Build history of the part. All positions in model axes, mm. A direction names the side the tool comes from. Coordinates: 2 decimals unless noted, no trailing zeros. Order: outer loops, then holes, each group sorted by start corner. A loop starts at its lowest first (then second) coordinate and runs counter-clockwise, first axis right, second up. Notation, with made-up numbers: (42.5, 69.25) - (76.5, 69.25) arc R28 ccw to (76.5, 106.25) - close; hole circle Ø2 at (2, -30.75). An arc over 180 degrees is marked (long way). Write each question's results on one line, items separated by ' | '.
Autodesk Inventor part; units mm, degrees
ref_plane "YZ Plane" through (0, 0, 0) normal (1, 0, 0) x (0, 1, 0)
ref_plane "XZ Plane" through (0, 0, 0) normal (0, 1, 0) x (-1, 0, 0)
ref_plane "XY Plane" through (0, 0, 0) normal (0, 0, 1) x (1, 0, 0)
sketch "Sketch1" plane through (0, 0, 0) normal (0, 1, 0) x (-1, 0, 0)
  circle A0 centre (0, 0) radius 2
  dimension "d0" = 4
extrude "Extrusion1" add sketch "Sketch1" along normal blind 35
sketch "Sketch2" plane through (0, 35, 0) normal (0, 1, 0) x (1, 0, 0)
  circle A0 centre (0, 0) radius 2
  circle A1 centre (0, 0) radius 3.5
  dimension "d3" = 7
extrude "Extrusion2" add sketch "Sketch2" along normal blind 4 contours A0 | A1
sketch "Sketch3" plane through (0, 39, 0) normal (0, 1, 0) x (1, 0, 0)
  circle A0 centre (0, 0) radius 3.5
  line L0 (0, 1.8475) -> (1.6, 0.9238)
  line L1 (1.6, 0.9238) -> (1.6, -0.9238)
  line L2 (1.6, -0.9238) -> (0, -1.8475)
  line L3 (0, -1.8475) -> (-1.6, -0.9238)
  line L4 (-1.6, -0.9238) -> (-1.6, 0.9238)
  line L5 (-1.6, 0.9238) -> (0, 1.8475)
  dimension "d6" = 1.6
extrude "Extrusion3" cut sketch "Sketch3" against normal blind 3 contours L0 L1 L2 L3 L4 L5
thread "Thread1"
chamfer "Chamfer1" distance 0.25 angle 45 1 edges at (2, 0, 0)
properties part number "SHCS4x35"
1. Tool access for faces 1 (the face through (2, 35, 2)), 2 (the face through (3.233, 36.972, -1.341)), 3 (the face through (0.81, 37.52, 1.38)): list every direction of +Z, -Z, +X, -X, +Y, -Y with a clear straight run to the whole face (end or side of a thin tool).
Solved:
face 1: -Y | face 2: +Y, -Y | face 3: +Y
2. Band-saw the part on C-C on x = -3. Give the cut face in (y, z).
Solved:
outline: (35, -1.8) - (39, -1.8) - (39, 1.8) - (35, 1.8) - close
3. Band-saw the part on B-B on y = 9. Give the cut face in (x, z).
Solved:
outline: circle Ø4 at (0, 0)
4. Probe line 1 (Y direction, x = -2.25, z = 1.5); line 2 (Z direction, x = -0.75, y = 11.5); line 3 (Y direction, x = -0.75, z = 1.25). List the from-to ranges inside material, lowest first.
Solved:
line 1: y = 35 to 39 | line 2: z = -1.85 to 1.85 | line 3: y = 0 to 36
5. Band-saw the part on D-D on x = 2.5. Give the cut face in (y, z).
Solved:
outline: (35, -2.45) - (39, -2.45) - (39, 2.45) - (35, 2.45) - close
6. Band-saw the part on A-A on z = 0. Give the cut face in (x, y).
Solved:
outline: (-3.5, 35) - (-2, 35) - (-2, 0.25) - (-1.75, 0) - (1.75, 0) - (2, 0.25) - (2, 35) - (3.5, 35) - (3.5, 39) - (1.6, 39) - (1.6, 36) - (-1.6, 36) - (-1.6, 39) - (-3.5, 39) - close
7. Drop flat-ended pins along their axis: pin 1 Ø1 at (y, z) = (32, -1.5) entering from +X; pin 2 Ø3 at (y, z) = (22, 2) entering from -X; pin 3 Ø1 at (x, z) = (-1, 0) entering from +Y. Give the stop position or say it passes through.
Solved:
pin 1: stops at x = 1.73 | pin 2: stops at x = -1.94 | pin 3: stops at y = 36
8. Two-plate mould, pull along Z, no slides. Class faces 4 (the face through (0, 17, 2)), 5 (the face through (0, 36, 0)), 6 (the face through (0, 0, 0)): +Z half, -Z half, draft (parallel to the pull), parting line (faces both ways), or undercut.
Solved:
face 4: parting line | face 5: undercut | face 6: draft
